Design review of the part built by this model. Coordinates are the model's own, in mm. Face numbers are marked on the shaded views. Give positions to 0.01 mm unless a question says otherwise; leave off trailing zeros. Write each loop counter-clockwise with the first axis right and the second up, starting at its lowest first coordinate (ties: lowest second). Pieces come first, ordered by that corner, then holes. Notation, with made-up numbers: (-25, 22) -> (11, 22) arc R22 cw to (11, 50) -> close; hole circle Ø9 at (18, 1.5). An arc over 180 degrees is marked (long way). Answer as a JSON object with one key per item and string values.
Autodesk Inventor part; units mm, degrees
ref_plane "Work Plane1" through (35, 0, 0) normal (-1, 0, 0) x (0, 0, 1)
ref_plane "Work Plane2" through (0, 15, 0) normal (0, 1, 0) x (1, 0, 0)
ref_plane "YZ Plane" through (0, 0, 0) normal (1, 0, 0) x (0, 1, 0)
sketch "Sketch1" plane through (0, 0, 0) normal (0, 0, 1) x (1, 0, 0)
  line L0 (0, 0) -> (70, 0)
  line L1 (70, 0) -> (70, 30)
  line L2 (70, 30) -> (0, 30)
  line L3 (0, 30) -> (0, 0)
  line L4 (55, 15) -> (55, 25)
  line L5 (55, 25) -> (35, 25)
  line L6 (68, 15) -> (68, 25)
  line L7 (68, 25) -> (60, 25)
  line L8 (60, 25) -> (60, 15)
  line L9 (15, 15) -> (15, 25)
  line L10 (15, 25) -> (35, 25)
  line L11 (2, 15) -> (2, 25)
  line L12 (2, 25) -> (10, 25)
  line L13 (10, 25) -> (10, 15)
  line L14 (55, 15) -> (55, 5)
  line L15 (55, 5) -> (35, 5)
  line L16 (68, 15) -> (68, 5)
  line L17 (68, 5) -> (60, 5)
  line L18 (60, 5) -> (60, 15)
  line L19 (15, 5) -> (35, 5)
  line L20 (15, 15) -> (15, 5)
  line L21 (10, 5) -> (10, 15)
  line L22 (2, 5) -> (10, 5)
  line L23 (2, 15) -> (2, 5)
  dimension "d0" = 70
  dimension "d1" = 30
  dimension "d2" = 20
  dimension "d3" = 10
  dimension "d5" = 8
extrude "Extrusion1" add sketch "Sketch1" against normal blind 10
sketch "Sketch2" plane through (0, 0, -10) normal (0, 0, -1) x (-1, 0, 0)
  line L0 (-70, 30) -> (-70, 0)
  line L1 (-70, 30) -> (0, 30)
  line L2 (0, 30) -> (0, 0)
  line L3 (0, 0) -> (-70, 0)
  line L4 (-70, 0) -> (-70, 30)
  line L5 (-68, 28) -> (-68, 2)
  line L6 (-2, 2) -> (-2, 28)
  line L7 (-68, 28) -> (-68, 30)
  line L8 (-70, 30) -> (0, 30)
  line L9 (-68, 2) -> (-68, 0)
  line L10 (-2, 2) -> (-2, 0)
  line L11 (-2, 28) -> (-2, 30)
  line L12 (-68, 30) -> (-2, 30)
  line L13 (-2, 30) -> (-2, 0)
  line L14 (-2, 0) -> (-68, 0)
  line L15 (-68, 0) -> (-68, 30)
extrude "Extrusion2" cut sketch "Sketch2" against normal blind 8 contours L1 L11 L6 L10 L3 L9 L5 L7
sketch "Sketch3" plane through (0, 30, 0) normal (0, 1, 0) x (1, 0, 0)
  line L0 (0, 10) -> (2, 10)
  circle A0 centre (1, 16.6661) radius 5
  circle A1 centre (1, 16.6661) radius 7
  point P0 (0, 0)
  dimension "d11" = 10
  dimension "d12" = 2
extrude "Extrusion3" add sketch "Sketch3" against normal blind 5
ref_plane "Work Plane1" through (35, 0, 0) normal (-1, 0, 0) x (0, 0, 1)
ref_plane "Work Plane2" through (0, 15, 0) normal (0, 1, 0) x (1, 0, 0)
mirror "Mirror1" about plane through (0, 15, 0) normal (0, 1, 0) of "Extrusion3"
mirror "Mirror2" about plane through (35, 0, 0) normal (-1, 0, 0) of "Extrusion3", "Mirror1"
properties part number "Slider 10mm"
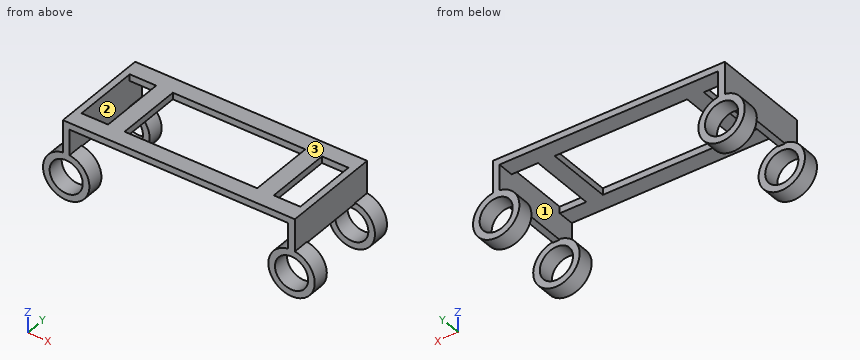
(1) For line 1 along Z through (x, y) = (69, 1.9); line 2 along X through (y, z) = (14.75, -1); line 3 along X through (y, z) = (28.5, -9.25), list the stretches that pass through material, from the lowest coordinate up.
Here are the results:
{"line 1": "z = -23.67 to -21.67, -11.67 to 0", "line 2": "x = 0 to 2, 10 to 15, 55 to 60, 68 to 70", "line 3": "x = 0 to 2, 68 to 70"}
(2) We need section B-B, the plane z = -5.5. State the section outline as (x, y) points, then the cut area to 3 significant figures.
Here are the results:
{"outline": "(0, 0) -> (2, 0) -> (2, 30) -> (0, 30) -> close; (68, 0) -> (70, 0) -> (70, 30) -> (68, 30) -> close", "area": "120 mm²"}
(3) We need section D-D, the plane y = 10. State the section outline as (x, z) points.
Here are the results:
{"outline": "(0, -10) -> (2, -10) -> (2, 0) -> (0, 0) -> close; (10, -2) -> (15, -2) -> (15, 0) -> (10, 0) -> close; (55, -2) -> (60, -2) -> (60, 0) -> (55, 0) -> close; (68, -10) -> (70, -10) -> (70, 0) -> (68, 0) -> close"}
(4) The part is to be moulded in two halves that separate along Y. For the marked faces 1, 2 and 3, say which applies: +Y half, -Y half, draft (parallel to the pull), parting line (faces both ways), or undercut.
Here are the results:
{"face 1": "undercut", "face 2": "undercut", "face 3": "draft"}
(5) We need section C-C, the plane x = 69. State the section outline as (y, z) points, then the cut area to 3 significant figures.
Here are the results:
{"outline": "(0, -23.67) -> (5, -23.67) -> (5, -21.67) -> (0, -21.67) -> close; (0, -11.67) -> (5, -11.67) -> (5, -10) -> (25, -10) -> (25, -11.67) -> (30, -11.67) -> (30, 0) -> (0, 0) -> close; (25, -23.67) -> (30, -23.67) -> (30, -21.67) -> (25, -21.67) -> close", "area": "337 mm²"}
(6) Clearance check with flat-ended pins moving along their axes: pin 1 (8 mm diameter, centred on y = 21.5, z = -2.5, fed in from -X); pin 2 (1 mm diameter, centred on x = 5.5, z = -1, fed in from -Y); pin 3 (1.6 mm diameter, centred on x = 68.5, y = 13, fed in from -Z); pin 4 (12 mm diameter, centred on y = 21.5, z = -6, fed in from -X). State where each tip first meets the part, or that it passes through.
Here are the results:
{"pin 1": "stops at x = 0", "pin 2": "stops at y = 0", "pin 3": "stops at z = -10", "pin 4": "stops at x = -2.93"}
(7) We need section A-A, the plane x = 49.5. State the section outline as (y, z) points.
Here are the results:
{"outline": "(0, -2) -> (5, -2) -> (5, 0) -> (0, 0) -> close; (25, -2) -> (30, -2) -> (30, 0) -> (25, 0) -> close"}
